Verification items for the finished model (mm, model axes). A direction names the side the tool comes from. Coordinates: 2 decimals unless noted, no trailing zeros. Loops run counter-clockwise (first coordinate to the right, second up) from the corner with the lowest first, then second, coordinate; pieces in that order, holes last. Notation, with made-up numbers: (50.25, 85.5) - (100.25, 85.5) arc R12 ccw to (100.25, 103.5) - close; hole circle Ø10 at (39, 2). An arc over 180 degrees is marked (long way). One line per item, written item: value. Start each with the question number.
(1) Gauge pin test, flat ends, axial feed: P1, Ø1.5, axis at y = -6.5, z = -1, coming from the -X side; P2, Ø1, axis at x = -21, z = 0, coming from the +Y side; P3, Ø5, axis at x = -21.5, y = -14, coming from the -Z side. Record the tip position at first contact, or that the pin passes through.
(2) Thickness scan on probe 1 along Z at (x, y) = (21, -15.5); probe 2 along Y at (x, z) = (-0.5, 0.3); probe 3 along X at (y, z) = (-18, -0.25). Record the ranges inside material, lowest first. Write a range as [from, to].
(3) Set-up check for faces 1 (the face through (23.846, 7.509, -1.047)), 2 (the face through (0, 0, 1)): record each of +Z, -Z, +X, -X, +Y, -Y from which the full face is reachable in a straight line by a thin tool's end or side.
(4) Section check A-A (x = 0). Record the boundary of the cut face in (y, z), plus the area to 3 significant figures.
```python
from build123d import *


with BuildPart() as f1:
    # F0 (on Front) → F1 (revolve)
    with BuildSketch(Plane.XZ):
        with BuildLine():
            Line((0, 1), (0, 0))
            Line((0, 0), (0, -2.866025))
            Line((0, -2.866025), (24.5, -2.866025))
            Line((24.5, -2.866025), (25.5, -1.866025))
            Line((25.5, -1.866025), (25, -1.866025))
            Line((25, -1.866025), (25, -1))
            Line((25, -1), (25, -0.25))
            ThreePointArc((25, -0.25), (25.073223, -0.073223), (25.25, 0))
            Line((25.25, 0), (28, 0))
            Line((28, 0), (28, 0.5))
            ThreePointArc((28, 0.5), (27.853553, 0.853553), (27.5, 1))
            Line((27.5, 1), (0, 1))
        make_face()
    revolve(axis=Axis((0, 0, -1.433013), (0, 0, 1)))


solid = f1.part
```
Responses:
1. P1: stops at x = -24.33
1. P2: stops at y = 19.07
1. P3: stops at z = -2.87
2. probe 1: z = [0, 1]
2. probe 2: y = [-28, 28]
2. probe 3: x = [-17.35, 17.35]
3. face 1: none
3. face 2: +Z, +X, -X, +Y, -Y
4. outline: (-28, 0) - (-25.25, 0) arc R0.25 cw to (-25, -0.25) - (-25, -1.87) - (-25.5, -1.87) - (-24.5, -2.87) - (24.5, -2.87) - (25.5, -1.87) - (25, -1.87) - (25, -0.25) arc R0.25 cw to (25.25, 0) - (28, 0) - (28, 0.5) arc R0.5 ccw to (27.5, 1) - (-27.5, 1) arc R0.5 ccw to (-28, 0.5) - close
4. area: 199 mm²
